Could you check a few things on this model? Use its own coordinates, in mm. Face numbers are marked on the shaded views. A direction names the side the tool comes from. Coordinates: 2 decimals unless noted, no trailing zeros. Order: outer loops, then holes, each group sorted by start corner. A loop starts at its lowest first (then second) coordinate and runs counter-clockwise, first axis right, second up. Notation, with made-up numbers: (12.5, 78.5) -> (18.5, 78.5) arc R15 ccw to (18.5, 87.5) -> close; hole circle Ø4 at (16.25, -22.75). An arc over 180 degrees is marked (long way). Use a Markdown table: item, result. Add a question column.
1) If we section it at D-D (y = -7.5): Write out the boundary of the cut face in (x, z).
2) Which directions (+Z, -Z, +X, -X, +Y, -Y) give clear straight access to the entire face, cutting with the end or side of a thin tool? Please do the marked faces 1 and 2.
3) Will this pin go through, and if not, where does the flat tip stop? pin 1 Ø1 at (y, z) = (-16, 4.5) entering from -X.
4) Thinking about a two-plate mould opening in X: for the marked faces 3, 4 and 5, which applies, +X half, -X half, draft (parallel to the pull), parting line (faces both ways), or undercut?
5) If we section it at C-C (x = -15.5): Write out the boundary of the cut face in (y, z), plus the area to 3 significant figures.
6) If we section it at B-B (z = 1.5): Write out the boundary of the cut face in (x, y), plus the area to 3 significant figures.
7) If I drill on L1, parallel to Y at x = 15.5, z = 5; L2, parallel to Y at x = 0, z = 4.25; L3, parallel to X at y = -5, z = 7.25, over which ranges is the centre line in solid material (lowest first)? Write a range as [from, to].
8) If we section it at A-A (y = -15.5): Write out the boundary of the cut face in (x, z), plus the area to 3 significant figures.
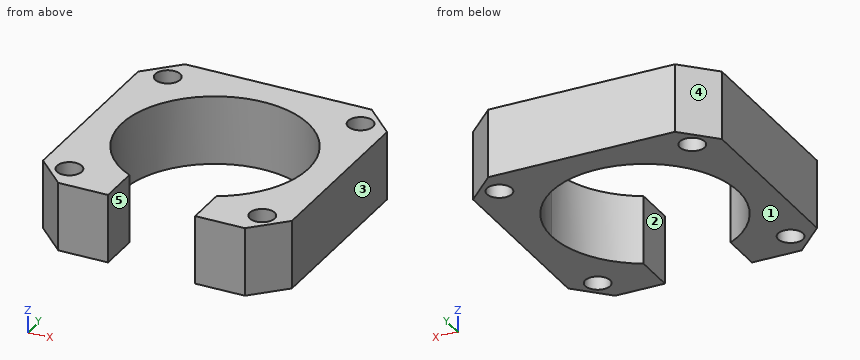
```python
from build123d import *

# Parameters (mm, degrees)
F0_R     = 2
F1_DEPTH = 11
F2_SIZE  = 5


with BuildPart() as f1:
    # F0 (on Top) → F1 (new body)
    with BuildSketch(Plane.XY):
        with BuildLine():
            Line((20, -20), (20, 20))
            Line((20, 20), (-20, 20))
            Line((-20, 20), (-20, -20))
            Line((-20, -20), (-7, -20))
            Line((-7, -20), (-7, -13.266499))
            ThreePointArc((-7, -13.266499), (-7.745967, 12.845233), (15, 0))
            ThreePointArc((15, 0), (12.845233, -7.745967), (7, -13.266499))
            Line((7, -13.266499), (7, -20))
            Line((7, -20), (20, -20))
        make_face()
        with Locations((-15.5, -15.5)):
            Circle(F0_R, mode=Mode.SUBTRACT)
        with Locations((15.5, -15.5)):
            Circle(F0_R, mode=Mode.SUBTRACT)
        with Locations((-15.5, 15.5)):
            Circle(F0_R, mode=Mode.SUBTRACT)
        with Locations((15.5, 15.5)):
            Circle(F0_R, mode=Mode.SUBTRACT)
    extrude(amount=F1_DEPTH)

    # F2
    f2_edges = [f1.edges().sort_by_distance(p)[0] for p in [
        (-20, -20, 5.5),
        (-20, 20, 5.5),
        (20, 20, 5.5),
        (20, -20, 5.5),
    ]]
    chamfer(f2_edges, length=F2_SIZE)


solid = f1.part
```
Answer sheet:
| question | item | result |
|---|---|---|
| 1 | outline | (-20, 0) -> (-12.99, 0) -> (-12.99, 11) -> (-20, 11) -> close; (12.99, 0) -> (20, 0) -> (20, 11) -> (12.99, 11) -> close |
| 2 | face 1 | -Z, +X, -X, +Y, -Y |
| 2 | face 2 | +Z, -Z, -Y |
| 3 | pin 1 | x = -19.5 |
| 4 | face 3 | +X half |
| 4 | face 4 | -X half |
| 4 | face 5 | undercut |
| 5 | outline | (-19.5, 0) -> (-17.5, 0) -> (-17.5, 11) -> (-19.5, 11) -> close; (-13.5, 0) -> (13.5, 0) -> (13.5, 11) -> (-13.5, 11) -> close; (17.5, 0) -> (19.5, 0) -> (19.5, 11) -> (17.5, 11) -> close |
| 5 | area | 341 mm2 |
| 6 | outline | (-20, -15) -> (-15, -20) -> (-7, -20) -> (-7, -13.27) arc R15 cw (long way) to (15, 0) arc R15 cw to (7, -13.27) -> (7, -20) -> (15, -20) -> (20, -15) -> (20, 15) -> (15, 20) -> (-15, 20) -> (-20, 15) -> close; hole circle Ø4 at (-15.5, -15.5); hole circle Ø4 at (-15.5, 15.5); hole circle Ø4 at (15.5, -15.5); hole circle Ø4 at (15.5, 15.5) |
| 6 | area | 715 mm2 |
| 7 | L1 | [-19.5, -17.5], [-13.5, 13.5], [17.5, 19.5] |
| 7 | L2 | [15, 20] |
| 7 | L3 | [-20, -14.14], [14.14, 20] |
| 8 | outline | (-19.5, 0) -> (-17.5, 0) -> (-17.5, 11) -> (-19.5, 11) -> close; (-13.5, 0) -> (-7, 0) -> (-7, 11) -> (-13.5, 11) -> close; (7, 0) -> (13.5, 0) -> (13.5, 11) -> (7, 11) -> close; (17.5, 0) -> (19.5, 0) -> (19.5, 11) -> (17.5, 11) -> close |
| 8 | area | 187 mm2 |
